The listing builds one solid part. Answer for the finished solid, in the listing's coordinates (mm). Face numbers are marked on the shaded views. Coordinates: 2 decimals unless noted, no trailing zeros. Write each loop counter-clockwise with the first axis right and the second up, starting at its lowest first coordinate (ties: lowest second). Pieces come first, ordered by that corner, then holes.
(1) The part is cut by section C-C on y = 82.5. Determine the outline of the cut face in (x, z), plus the area to 3 significant figures.
(2) The part is cut by section D-D on z = -32.5. Determine the outline of the cut face in (x, y), plus the area to 3 significant figures.
(3) The part is cut by section B-B on z = 0. Determine the outline of the cut face in (x, y).
(4) Given P1, Ø2, axis at x = 22, y = 227, coming from the +Z side; P2, Ø10, axis at x = -20.5, y = 103, coming from the +Z side; P3, Ø6, axis at y = 351.5, z = -11.5, coming from the +X side, each flat-ended and moving along its own axis, determine where each tip first touches the part or whether it passes through.
(5) The part is cut by section A-A on x = 0. Determine the outline of the cut face in (y, z).
(6) Straight lines are drawn through the part: line 1 (Z direction, x = 1.5, y = 347); line 2 (X direction, y = 11, z = -14.5); line 3 (X direction, y = 280.5, z = -16). For each, find the intervals that lie inside material, in ascending order.
(7) For a pull along X with two mould halves and no side action, classify the marked faces 1 and 2 as +X half, -X half, draft (parallel to the pull), parting line (faces both ways), or undercut.
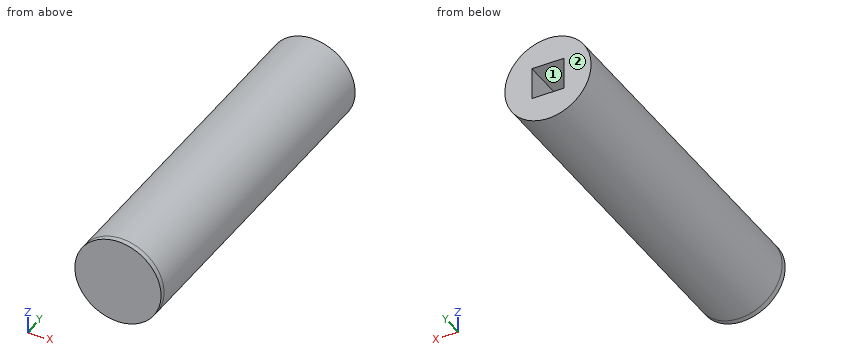
from build123d import *

# Parameters (mm, degrees)
SKETCH1_R           = 51.1302
SKETCH1_W           = 38.1
SKETCH1_H           = 38.1
BOSS_EXTRUDE1_DEPTH = 406.4
BOSS_EXTRUDE2_START = 6.35
SKETCH2_R           = 51.1302
BOSS_EXTRUDE2_DEPTH = 6.35


with BuildPart() as part:
    # Sketch1 → Boss-Extrude1 (new body)
    with BuildSketch(Plane(origin=(0, 0, 0), x_dir=(1, 0, 0), z_dir=(0, 1, 0))):
        with Locations(Location((0, 0, 0), (0, 0, 270))):
            Circle(SKETCH1_R)
        Rectangle(SKETCH1_W, SKETCH1_H, mode=Mode.SUBTRACT)
    extrude(amount=BOSS_EXTRUDE1_DEPTH)

    # Sketch2 → Boss-Extrude2 (add)
    with BuildSketch(Plane.XZ.offset(BOSS_EXTRUDE2_START)):
        with Locations(Location((0, 0, 0), (0, 0, 270))):
            Circle(SKETCH2_R)
    extrude(amount=-BOSS_EXTRUDE2_DEPTH)


solid = part.part
Model answer:
1. outline: circle Ø102.26 at (0, 0); hole (-19.05, -19.05) - (19.05, -19.05) - (19.05, 19.05) - (-19.05, 19.05) - close
1. area: 6,760 mm2
2. outline: (-39.47, -6.35) - (39.47, -6.35) - (39.47, 406.4) - (-39.47, 406.4) - close
2. area: 32,600 mm2
3. outline: (-51.13, -6.35) - (51.13, -6.35) - (51.13, 406.4) - (19.05, 406.4) - (19.05, 0) - (-19.05, 0) - (-19.05, 406.4) - (-51.13, 406.4) - close
4. P1: stops at z = 46.62
4. P2: stops at z = 48.72
4. P3: stops at x = 50.42
5. outline: (-6.35, -51.13) - (406.4, -51.13) - (406.4, -19.05) - (0, -19.05) - (0, 19.05) - (406.4, 19.05) - (406.4, 51.13) - (-6.35, 51.13) - close
6. line 1: z = -51.11 to -19.05, 19.05 to 51.11
6. line 2: x = -49.03 to -19.05, 19.05 to 49.03
6. line 3: x = -48.56 to -19.05, 19.05 to 48.56
7. face 1: undercut
7. face 2: draft
